Part model, mm, in its own coordinate system. A direction names the side the tool comes from. Give positions to 0.01 mm unless a question says otherwise; leave off trailing zeros. Loops run counter-clockwise (first coordinate to the right, second up) from the corner with the lowest first, then second, coordinate; pieces in that order, holes last. Notation, with made-up numbers: M 29,-11.5 L 57,-11.5 A13 ccw 57,11.5 Z; hole C -11.5,64.5 d2. An arc over 180 degrees is marked long. Answer in a Markdown table with one row per item.
from build123d import *

# Parameters (mm, degrees)
SKETCH1_R           = 35.75
BOSS_EXTRUDE1_DEPTH = 2
BOSS_EXTRUDE2_DEPTH = 22
SKETCH3_W           = 29.5
SKETCH3_H           = 35
BOSS_EXTRUDE3_DEPTH = 10
SKETCH4_R           = 1.4
SKETCH4_R_2         = 1.25
CUT_EXTRUDE1_DEPTH  = 2
CUT_EXTRUDE2_DEPTH  = 10
SKETCH6_R           = 1.7
CUT_EXTRUDE3_DEPTH  = 34
CUT_EXTRUDE4_DEPTH  = 10


with BuildPart() as part:
    # Sketch1 → Boss-Extrude1 (new body)
    with BuildSketch(Plane.XY):
        Circle(SKETCH1_R)
    extrude(amount=BOSS_EXTRUDE1_DEPTH)

    # Sketch2 → Boss-Extrude2 (add)
    with BuildSketch(Plane(origin=(0, 0, 0), x_dir=(-1, 0, 0), z_dir=(0, 0, -1))):
        Polygon((14.75, 26), (-14.75, 26), (-14.75, -9), (-15.55, -9), (-15.55, 26.8), (15.55, 26.8), (15.55, -9), (14.75, -9), align=None)
    extrude(amount=BOSS_EXTRUDE2_DEPTH)

    # Sketch3 → Boss-Extrude3 (add)
    with BuildSketch(Plane(origin=(0, 0, 0), x_dir=(-1, 0, 0), z_dir=(0, 0, -1))):
        with Locations((0, 8.5)):
            Rectangle(SKETCH3_W, SKETCH3_H)
    extrude(amount=BOSS_EXTRUDE3_DEPTH)

    # Sketch4 → Cut-Extrude1 (cut)
    with BuildSketch(Plane.XZ.offset(-26)):
        with Locations((-11.25, -13.5)):
            Circle(SKETCH4_R)
        with Locations((11.25, -13.5)):
            Circle(SKETCH4_R_2)
    extrude(amount=-CUT_EXTRUDE1_DEPTH, mode=Mode.SUBTRACT)

    # Sketch5 → Cut-Extrude2 (cut)
    with BuildSketch(Plane.XY.offset(2)):
        Polygon((-17.5, 12), (-23.5, 12), (-23.5, 22.131751807), (-17.5, 22), align=None)
    extrude(amount=-CUT_EXTRUDE2_DEPTH, mode=Mode.SUBTRACT)

    # Sketch6 → Cut-Extrude3 (cut)
    with BuildSketch(Plane.XY.offset(2)):
        with Locations((0, 31)):
            Circle(SKETCH6_R)
        with Locations((-31, 0)):
            Circle(SKETCH6_R)
        with Locations((31, 0)):
            Circle(SKETCH6_R)
        with Locations((0, -31)):
            Circle(SKETCH6_R)
    extrude(amount=-CUT_EXTRUDE3_DEPTH, mode=Mode.SUBTRACT)

    # Sketch7 → Cut-Extrude4 (cut)
    with BuildSketch(Plane.XY.offset(2)):
        Polygon((-17.5, 12), (-23.5, 12), (-23.5, 35.926459787), (-17.5, 35.79470798), align=None)
    extrude(amount=-CUT_EXTRUDE4_DEPTH, mode=Mode.SUBTRACT)


solid = part.part
(1) Which spindle directions (+Z, -Z, +X, -X, +Y, -Y) get a long thin tool onto all of the face, cutting with end or side? Do faces 1 (the face through (-14.75, 8, -16)), 2 (the face through (-23.5, 19, 1)), 3 (the face through (15.55, 9, -11)). Say none if no direction does.
Recorded:
| item | result |
|---|---|
| face 1 | -Z, -Y |
| face 2 | +Z, -Z, +Y |
| face 3 | -Z, +X, +Y, -Y |
(2) Saw through at A-A (z = -13.5). Write the cut outline in (x, y).
Recorded:
| item | result |
|---|---|
| outline | M -15.55,-9 L -14.75,-9 L -14.75,26 L -12.65,26 L -12.65,26.8 L -15.55,26.8 Z; M -9.85,26 L 10,26 L 10,26.8 L -9.85,26.8 Z; M 12.5,26 L 14.75,26 L 14.75,-9 L 15.55,-9 L 15.55,26.8 L 12.5,26.8 Z |
(3) Pin check, flat tips, straight feed: pin 1 Ø3 at (x, z) = (11.25, -13.5) entering from +Y; pin 2 Ø23.5 at (x, y) = (1, 2.5) entering from -Z; pin 3 Ø6 at (y, z) = (6.5, -18) entering from +X; pin 4 Ø21.5 at (x, y) = (-12, 16) entering from -Z. Stop position of each tip, or through.
Recorded:
| item | result |
|---|---|
| pin 1 | stops at y = 26.8 |
| pin 2 | stops at z = -10 |
| pin 3 | stops at x = 15.55 |
| pin 4 | stops at z = -22 |
(4) Drill centre lines: line 1 along Y through (x, z) = (0, 1.1); line 2 along X through (y, z) = (16.5, -15.75); line 3 along Z through (x, y) = (25, -2). Where is each one in solid material? Low to high.
Recorded:
| item | result |
|---|---|
| line 1 | y = -35.75 to -32.7, -29.3 to 29.3, 32.7 to 35.75 |
| line 2 | x = -15.55 to -14.75, 14.75 to 15.55 |
| line 3 | z = 0 to 2 |
(5) Saw through at D-D (y = 13.5). Write the cut outline in (x, z).
Recorded:
| item | result |
|---|---|
| outline | M -33.1,0 L -23.5,0 L -23.5,2 L -33.1,2 Z; M -17.5,0 L -15.55,0 L -15.55,-22 L -14.75,-22 L -14.75,-10 L 14.75,-10 L 14.75,-22 L 15.55,-22 L 15.55,0 L 33.1,0 L 33.1,2 L -17.5,2 Z |
(6) Saw through at B-B (x = -31). Write the cut outline in (y, z).
Recorded:
| item | result |
|---|---|
| outline | M -17.81,0 L -1.7,0 L -1.7,2 L -17.81,2 Z; M 1.7,0 L 17.81,0 L 17.81,2 L 1.7,2 Z |
(7) Saw through at C-C (y = 0). Write the cut outline in (x, z), plus the area to 3 significant figures.
Recorded:
| item | result |
|---|---|
| outline | M -35.75,0 L -32.7,0 L -32.7,2 L -35.75,2 Z; M -29.3,0 L -15.55,0 L -15.55,-22 L -14.75,-22 L -14.75,-10 L 14.75,-10 L 14.75,-22 L 15.55,-22 L 15.55,0 L 29.3,0 L 29.3,2 L -29.3,2 Z; M 32.7,0 L 35.75,0 L 35.75,2 L 32.7,2 Z |
| area | 460 mm^2 |
(8) Pull direction Z, two halves, no side cores. Call faces 4 (the face through (-12.28, 26.39, -12.55)), 5 (the face through (-1, -15, 0)), 6 (the face through (0, 26.8, -11)): +Z half, -Z half, draft (parallel to the pull), parting line (faces both ways), or undercut.
Recorded:
| item | result |
|---|---|
| face 4 | undercut |
| face 5 | -Z half |
| face 6 | draft |
